from build123d import *

# Parameters (mm, degrees)
F0_W     = 63.5
F0_H     = 63.5
F1_DEPTH = 50.8
F4_DEPTH = 2.032
F2_W     = 1.5281873676
F2_H     = 5.9584317987
F5_DEPTH = 8.382
F6_F1_R  = 3.175
F6_F2_R  = 3.175
F6_F3_R  = 3.175
F6_F4_R  = 3.175
F6_F5_R  = 3.175


with BuildPart() as f1:
    # F0 (on Top) → F1 (new body)
    with BuildSketch(Plane.XY):
        Rectangle(F0_W, F0_H)
    extrude(amount=F1_DEPTH)

    # F3 (on face) → F4 (cut)
    with BuildSketch(Plane.XY.offset(50.8)):
        with BuildLine():
            Line((-31.75, -13.081), (12.7, -13.081))
            ThreePointArc((12.7, -13.081), (25.781, 0), (12.7, 13.081))
            Line((12.7, 13.081), (-31.75, 13.081))
            Line((-31.75, 13.081), (-31.75, -13.081))
        make_face()
        Polygon((12.7063958977, -7.552316163), (6.1627002943, -3.7816970914), (6.1563043966, 3.7706190716), (12.6936041023, 7.552316163), (19.2372997057, 3.7816970914), (19.2436956034, -3.7706190716), align=None, mode=Mode.SUBTRACT)
    extrude(amount=-F4_DEPTH, mode=Mode.SUBTRACT)

    # F2 (on face) → F5 (cut)
    with BuildSketch(Plane.XY.offset(50.8)):
        with Locations((145.2675004168, 51.4206579864)):
            Rectangle(F2_W, F2_H)
        Polygon((12.6936041023, 7.552316163), (6.1563043966, 3.7706190716), (6.1627002943, -3.7816970914), (12.7063958977, -7.552316163), (19.2436956034, -3.7706190716), (19.2372997057, 3.7816970914), align=None)
    extrude(amount=-F5_DEPTH, mode=Mode.SUBTRACT)

    # F6: fillet of radius 3.175 on 13 edges, made by hand

    # F6_f1
    f6_f1_edges = [f1.edges().sort_by_distance(p)[0] for p in [
        (-31.75, 0, 0),
    ]]
    fillet(f6_f1_edges, radius=F6_F1_R)

    # F6_f2
    f6_f2_edges = [f1.edges().sort_by_distance(p)[0] for p in [
        (-31.75, -31.75, 26.9875),
    ]]
    fillet(f6_f2_edges, radius=F6_F2_R)

    # F6_f3
    f6_f3_edges = [f1.edges().sort_by_distance(p)[0] for p in [
        (-31.75, -20.828, 50.8),
    ]]
    fillet(f6_f3_edges, radius=F6_F3_R)

    # F6_f4
    f6_f4_edges = [f1.edges().sort_by_distance(p)[0] for p in [
        (-31.75, 31.75, 25.4),
    ]]
    fillet(f6_f4_edges, radius=F6_F4_R)

    # F6_f5
    f6_f5_edges = [f1.edges().sort_by_distance(p)[0] for p in [
        (31.75, 0, 0),
    ]]
    fillet(f6_f5_edges, radius=F6_F5_R)


solid = f1.part
Model file for the job. Use its own axes, mm. A direction names the side the tool comes from. Give positions to 0.01 mm unless a question says otherwise; leave off trailing zeros. Loops run counter-clockwise (first coordinate to the right, second up) from the corner with the lowest first, then second, coordinate; pieces in that order, holes last.
Item 1: Drop flat-ended pins along their axis: P1, Ø1.5, axis at x = 17.5, y = -2.5, coming from the +Z side; P2, Ø8, axis at x = 8.5, y = -3.5, coming from the +Z side; P3, Ø2, axis at x = -12, z = 50, coming from the -Y side. Give the stop position or say it passes through.
Check values:
P1: stops at z = 42.42
P2: stops at z = 48.77
P3: stops at y = -31.44
Item 2: Which spindle directions (+Z, -Z, +X, -X, +Y, -Y) get a long thin tool onto all of the face, cutting with end or side? Do faces 1 (the face through (-10, -13.081, 50)), 2 (the face through (0.4, 30.8, 49.89)), 3 (the face through (13, 0, 42.418)). Say none if no direction does.
Check values:
face 1: +Z, -X
face 2: +Z, +X, -X, +Y
face 3: +Z
Item 3: Slice it at B-B (y = 9). Write the cut outline in (x, z) (3 decimals), plus the area to 3 significant figures.
Check values:
outline: (-31.75, 3.175) arc R3.175 ccw to (-28.575, 0) - (28.575, 0) arc R3.175 ccw to (31.75, 3.175) - (31.75, 47.625) arc R3.175 ccw to (28.575, 50.8) - (22.193, 50.8) - (22.193, 48.768) - (-31.537, 48.768) arc R3.175 ccw to (-31.75, 47.625) - close
area: 3,110 mm2
Item 4: Slice it at A-A (x = 1). Write the cut outline in (y, z) (3 decimals).
Check values:
outline: (-31.75, 3.175) arc R3.175 ccw to (-28.575, 0) - (28.575, 0) arc R3.175 ccw to (31.75, 3.175) - (31.75, 47.625) arc R3.175 ccw to (28.575, 50.8) - (13.081, 50.8) - (13.081, 48.768) - (-13.081, 48.768) - (-13.081, 50.8) - (-28.575, 50.8) arc R3.175 ccw to (-31.75, 47.625) - close
Item 5: Mould opens along Y. For faces 4 (the face through (15.929, -5.688, 45.637)), 5 (the face through (-31.75, 0, 25)), 6 (the face through (-30.84, -30.8, 25.71)) say: +Y half, -Y half, draft (parallel to the pull), parting line (faces both ways), or undercut.
Check values:
face 4: undercut
face 5: draft
face 6: -Y half
Item 6: Drill centre lines: line 1 along Z through (x, y) = (19.5, -3.5); line 2 along Z through (x, y) = (9, -2.5); line 3 along Y through (x, z) = (-0.5, 3). Where is each one in solid material? Low to high.
Check values:
line 1: z = 0 to 48.77
line 2: z = 0 to 42.42
line 3: y = -31.75 to 31.75
